```python
from build123d import *

# Parameters (mm, degrees)
F0_W     = 6.216531
F0_H     = 6.35
F0_W_2   = 6.35
F0_W_3   = 11.1125
F0_H_2   = 7.46389
F2_R     = 3.96875
F3_DEPTH = 28.576


with BuildPart() as f1:
    # F0 (on Front) → F1 (revolve)
    with BuildSketch(Plane.XZ):
        with Locations((-24.436133, -7.781217)):
            Rectangle(F0_W, F0_H)
        Polygon((-18.152868, 7.063228), (-18.152868, 17.618783), (-21.327868, 17.618783), (-21.327868, 11.268783), (-21.327868, -4.606217), (-21.327868, -10.956217), (-18.152868, -10.956217), (-18.152868, -0.400662), align=None)
        with Locations((-24.502868, 14.443783)):
            Rectangle(F0_W_2, F0_H)
        with Locations((-12.596618, 3.331283)):
            Rectangle(F0_W_3, F0_H_2)
        Polygon((-7.040368, 17.618783), (-7.040368, 7.063228), (-7.040368, -0.400662), (-7.040368, -10.956217), (4.072132, -10.956217), (4.072132, 17.618783), align=None)
    revolve(axis=Axis((4.072132, 0, 3.331283), (0, 0, -1)))

    # F2 (on face) → F3 (cut, through all)
    with BuildSketch(Plane.XY.offset(17.618783)):
        with Locations((4.072132, 0)):
            Circle(F2_R)
    extrude(amount=-F3_DEPTH, mode=Mode.SUBTRACT)


solid = f1.part
```
The model under review builds one solid part; all positions refer to its coordinate system, in mm. A direction names the side the tool comes from. Round coordinates to 2 decimals unless told otherwise and drop trailing zeros. Loops run counter-clockwise (first coordinate to the right, second up) from the corner with the lowest first, then second, coordinate; pieces in that order, holes last. Notation, with made-up numbers: (47, -28) -> (80, -28) arc R21 cw to (80, 10) -> close; hole circle Ø5 at (45, 52). An arc over 180 degrees is marked (long way). Answer as a JSON object with one key per item and string values. Group by question number.
1) Mouldability with a two-part tool opening along Z and no side actions: class faces 1 (the face through (-17.127, 6.676, 12.415)), 2 (the face through (9, 0, 17.619)), 3 (the face through (18.3, 21.3, 11.269)), 4 (the face through (4, 26, -4.606)) as released by +Z, released by -Z, zero draft, split by the parting line, or undercut.
2) For faces 5 (the face through (0.92, -2.41, 3.53)), 6 (the face through (14.3, 5.3, 7.063)), 7 (the face through (-20.155, 7.629, 3.22)), 8 (the face through (-18, -7, 17.619)), 9 (the face through (14.3, 5.3, -0.401)), list the 3-axis set-ups (+Z, -Z, +X, -X, +Y, -Y) from which the entire face can be reached by the end or side of a thin tool; tool diameter is ignored.
3) We need section D-D on y = 14.5. Write out the cut boundary in (x, z).
4) We need section A-A on z = 8. Give the number of separate pieces and of enclosed holes in the cut face, then the cut area to 3 significant figures.
5) For pin 1 Ø1.5 at (x, z) = (2, -4.5) entering from +Y; pin 2 Ø5 at (x, y) = (4.07, 0) entering from +Z; pin 3 Ø8 at (x, z) = (7.5, 2.5) entering from +Y; pin 4 Ø5 at (y, z) = (-5.5, -7.5) entering from -X, all flat-tipped, find the tip position at first contact; note any pin that passes through.
6) For line 1 (X direction, y = 10, z = -8.75); line 2 (Z direction, x = 17, y = 28); line 3 (Y direction, x = 14, z = -9.75), list the stretches that pass through material, from the lowest coordinate up. Write a range as [from, to].
Result set:
{
 "1": {"face 1": "zero draft", "face 2": "released by +Z", "face 3": "undercut", "face 4": "undercut"},
 "2": {"face 5": "+Z, -Z", "face 6": "+Z", "face 7": "none", "face 8": "+Z, +X, -X, +Y, -Y", "face 9": "-Z"},
 "3": {"outline": "(-24.17, 11.27) -> (-16.78, 11.27) -> (-16.78, -4.61) -> (-24.02, -4.61) -> (-24.02, -10.96) -> (-12.77, -10.96) -> (-12.77, -0.4) -> (20.92, -0.4) -> (20.92, -10.96) -> (32.17, -10.96) -> (32.17, -4.61) -> (24.93, -4.61) -> (24.93, 11.27) -> (32.32, 11.27) -> (32.32, 17.62) -> (20.92, 17.62) -> (20.92, 7.06) -> (-12.77, 7.06) -> (-12.77, 17.62) -> (-24.17, 17.62) -> close"},
 "4": {"separate pieces": "2", "enclosed holes": "2", "area": "814 mm²"},
 "5": {"pin 1": "y = 31.59", "pin 2": "through", "pin 3": "y = 25.4", "pin 4": "x = -27.4"},
 "6": {"line 1": "[-25.92, -15.78], [-0.77, 8.92], [23.92, 34.07]", "line 2": "[-10.96, -4.61], [11.27, 17.62]", "line 3": "[-30.02, -19.88], [-4.99, 4.99], [19.88, 30.02]"}
}
